Here's the drawing with two shaded views (mm, measured from the low corner). I have some questions. A direction names the side the tool comes from. Round coordinates to 2 decimals unless told otherwise and drop trailing zeros. Order: outer loops, then holes, each group sorted by start corner. A loop starts at its lowest first (then second) coordinate and runs counter-clockwise, first axis right, second up.
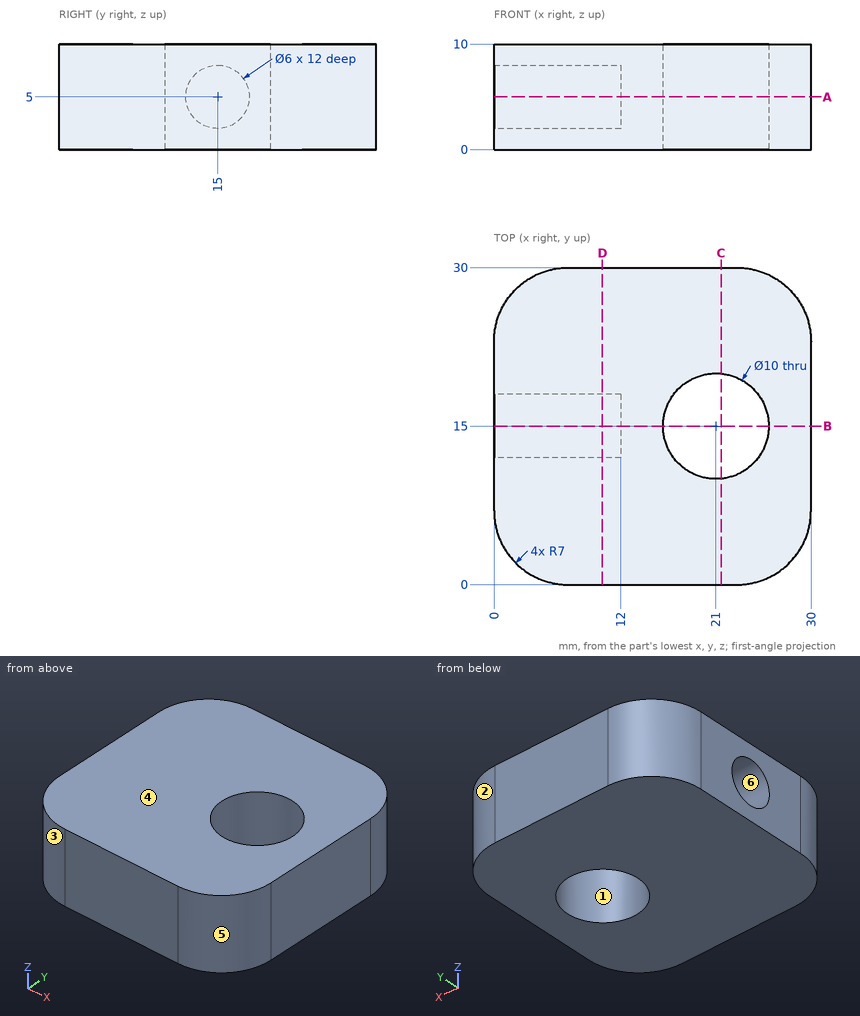
1. If we section it at D-D, the plane x = 10.25: Write out the boundary of the cut face in (y, z).
Evaluation:
outline: (0, 0) - (30, 0) - (30, 10) - (0, 10) - close; hole circle Ø6 at (15, 5)
2. I need wall thicknesses on probe 1 along Y at (x, z) = (21, 8); probe 2 along Y at (x, z) = (6.75, 5); probe 3 along X at (y, z) = (19.5, 8.25). Which ranges of each line are inside material? Lowest first, please.
Evaluation:
probe 1: y = 0 to 10, 20 to 30
probe 2: y = 0 to 12, 18 to 30
probe 3: x = 0 to 18.82, 23.18 to 30
3. If we section it at A-A, the plane z = 5: Write out the boundary of the cut face in (x, y).
Evaluation:
outline: (0, 7) arc R7 ccw to (7, 0) - (23, 0) arc R7 ccw to (30, 7) - (30, 23) arc R7 ccw to (23, 30) - (7, 30) arc R7 ccw to (0, 23) - (0, 18) - (12, 18) - (12, 12) - (0, 12) - close; hole circle Ø10 at (21, 15)
4. I'm going to push a flat-ended pin straight in: P1, Ø1.5, axis at x = 4, z = 6, coming from the +Y side. Where does the tip first touch, or does it pass through?
Evaluation:
P1: stops at y = 29.63
5. On a 3-axis mill with a long thin cutter (end or side, diameter ignored), from which of +Z, -Z, +X, -X, +Y, -Y can I reach the whole of each face in a straight line? I mean the marked faces 5 and 6. Say none if no direction works.
Evaluation:
face 5: +Z, -Z, +X, -Y
face 6: -X
6. If we section it at B-B, the plane y = 15: Write out the boundary of the cut face in (x, z), and give its area (3 significant figures).
Evaluation:
outline: (0, 0) - (16, 0) - (16, 10) - (0, 10) - (0, 8) - (12, 8) - (12, 2) - (0, 2) - close; (26, 0) - (30, 0) - (30, 10) - (26, 10) - close
area: 128 mm2
7. If we mould it in two halves opening along Y, with no side actions, what happens to the marked faces 1, 2, 3 and 4? For each: released by +Y, released by -Y, zero draft, split by the parting line, or undercut.
Evaluation:
face 1: undercut
face 2: released by +Y
face 3: released by -Y
face 4: zero draft
8. If we section it at C-C, the plane x = 21.5: Write out the boundary of the cut face in (y, z), and give its area (3 significant figures).
Evaluation:
outline: (0, 0) - (10.03, 0) - (10.03, 10) - (0, 10) - close; (19.97, 0) - (30, 0) - (30, 10) - (19.97, 10) - close
area: 201 mm2
